Here's how the part is built. I have some questions about the finished solid (model axes, mm). Round coordinates to 2 decimals unless told otherwise and drop trailing zeros. Write each loop counter-clockwise with the first axis right and the second up, starting at its lowest first coordinate (ties: lowest second). Pieces come first, ordered by that corner, then holes. Notation, with made-up numbers: M -34,5 L -9,5 A26 cw -9,38 Z; hole C 88,11.5 d2. An arc over 180 degrees is marked long. Use one line per item in the form item = value. Start each with the question number.
Q1. I need wall thicknesses on line 1 along Y through (x, z) = (0, 0.9); line 2 along X through (y, z) = (52.5, 1.1); line 3 along Y through (x, z) = (-25.4, 1.2). Which ranges of each line are inside material? Lowest first, please. Write a range as from..to.
Q2. I want a section at D-D on x = -21.5. List the corners of the cut face in (y, z) for me.
Q3. I want a section at C-C on y = 25.4. List the corners of the cut face in (x, z) for me, and give its area (3 significant figures).
Q4. I'm going to push flat-ended pins straight in: pin 1 Ø3 at (x, y) = (-51.3, -16.8) entering from +Z; pin 2 Ø1 at (x, z) = (-5, 0.5) entering from -Y. Where does each tip first touch, or does it pass through?
Q5. We'd pull the mould along X, two halves only. Please class faces 1 (the face through (57.095, -2.513, 1.628)), 2 (the face through (-2.82, 20.97, 1.63)), 3 (the face through (1, -1, 3.302)): +X half, -X half, draft (parallel to the pull), parting line (faces both ways), or undercut.
Q6. I want a section at A-A on y = 0. List the corners of the cut face in (x, z) for me.
```python
from build123d import *

# Parameters (mm, degrees)
SKETCH_1_R                     = 57.15
EXTRUDE_1_DEPTH                = 3.302
SKETCH_2_R                     = 1.651
CUT_EXTRUDE_1_DEPTH            = 81.889728668
M10_CLEARANCE_HOLE1_AT_2_COUNT = 2
M10_CLEARANCE_HOLE1_AT_2_PITCH = 50.8
CIRPATTERN1_COUNT              = 4


with BuildPart() as part:
    # 草图1 → 凸台-拉伸1 (new body)
    with BuildSketch(Plane.XY):
        with Locations(Location((0, 0, 0), (0, 0, 180))):
            Circle(SKETCH_1_R)
    extrude(amount=EXTRUDE_1_DEPTH)

    # 草图2 → 切除-拉伸1 (cut, through all)
    with BuildSketch(Plane(origin=(0, 0, 0), x_dir=(-1, 0, 0), z_dir=(0, 0, -1))):
        with Locations((-51.295425161, 16.7952369)):
            Circle(SKETCH_2_R)
        with Locations((-11.102610763, 52.820759738)):
            Circle(SKETCH_2_R)
        with Locations((40.192814398, 36.025522838)):
            Circle(SKETCH_2_R)
        with Locations((51.295425161, -16.7952369)):
            Circle(SKETCH_2_R)
        with Locations((11.102610763, -52.820759738)):
            Circle(SKETCH_2_R)
        with Locations((-40.192814398, -36.025522838)):
            Circle(SKETCH_2_R)
    extrude(amount=-CUT_EXTRUDE_1_DEPTH, mode=Mode.SUBTRACT)

    # Sketch3 → M10 Clearance Hole1 (revolve, cut)
    with BuildSketch(Plane.YZ.offset(25.4)):
        Polygon((0, 0), (0, 28.55451825), (5.25, 25.4), (5.25, 0), align=None)
    m10_clearance_hole1 = revolve(axis=Axis((25.4, 0, -6.35), (0, 0, 1)), mode=Mode.SUBTRACT)

    # M10 Clearance Hole1 at 2: M10 Clearance Hole1 ×2
    with Locations(*[(-i * M10_CLEARANCE_HOLE1_AT_2_PITCH, 0, 0) for i in range(1, M10_CLEARANCE_HOLE1_AT_2_COUNT)]):
        add(m10_clearance_hole1, mode=Mode.SUBTRACT)

    # CirPattern1: M10 Clearance Hole1 ×4 about axis
    cirpattern1_axis = Axis((0, 0, 0), (0, 0, 1))
    for i in range(1, CIRPATTERN1_COUNT):
        add(m10_clearance_hole1.rotate(cirpattern1_axis, i * 360 / CIRPATTERN1_COUNT), mode=Mode.SUBTRACT)

    # CirPattern1 copy 1 sketch → CirPattern1 copy 1 (revolve, cut)
    with BuildSketch(Plane(origin=(0, -25.4, 0), x_dir=(-1, 0, 0), z_dir=(0, 1, 0))):
        Polygon((0, 0), (0, 28.55451825), (5.25, 25.4), (5.25, 0), align=None)
    revolve(axis=Axis((0, -25.4, -6.35), (0, 0, 1)), mode=Mode.SUBTRACT)

    # CirPattern1 copy 2 sketch → CirPattern1 copy 2 (revolve, cut)
    with BuildSketch(Plane(origin=(25.4, 0, 0), x_dir=(0, -1, 0), z_dir=(-1, 0, 0))):
        Polygon((0, 0), (0, 28.55451825), (5.25, 25.4), (5.25, 0), align=None)
    revolve(axis=Axis((25.4, 0, -6.35), (0, 0, 1)), mode=Mode.SUBTRACT)

    # CirPattern1 copy 3 sketch → CirPattern1 copy 3 (revolve, cut)
    with BuildSketch(Plane.XZ.offset(-25.4)):
        Polygon((0, 0), (0, 28.55451825), (5.25, 25.4), (5.25, 0), align=None)
    revolve(axis=Axis((0, 25.4, -6.35), (0, 0, 1)), mode=Mode.SUBTRACT)


solid = part.part
```
Reported:
q1.line_1 = -57.15..-30.65, -20.15..20.15, 30.65..57.15
q1.line_2 = -22.58..9.48, 12.72..22.58
q1.line_3 = -51.2..-5.25, 5.25..51.2
q2.outline = M -52.95,0 L -3.51,0 L -3.51,3.3 L -52.95,3.3 Z; M 3.51,0 L 52.95,0 L 52.95,3.3 L 3.51,3.3 Z
q3.outline = M -51.2,0 L -5.25,0 L -5.25,3.3 L -51.2,3.3 Z; M 5.25,0 L 51.2,0 L 51.2,3.3 L 5.25,3.3 Z
q3.area = 303 mm^2
q4.pin_1 = through
q4.pin_2 = -56.97
q5.face_1 = parting line
q5.face_2 = undercut
q5.face_3 = draft
q6.outline = M -57.15,0 L -30.65,0 L -30.65,3.3 L -57.15,3.3 Z; M -20.15,0 L 20.15,0 L 20.15,3.3 L -20.15,3.3 Z; M 30.65,0 L 57.15,0 L 57.15,3.3 L 30.65,3.3 Z
